Study the drawing (mm; zero at the part's minimum x, y, z) and answer. Coordinates: 2 decimals unless noted, no trailing zeros. Order: outer loops, then holes, each group sorted by start corner. A loop starts at its lowest first (then second) coordinate and runs counter-clockwise, first axis right, second up. Notation, with made-up numbers: (-3, 23) - (45, 23) arc R19 ccw to (45, 46) - close; hole circle Ø5 at (18, 55). An arc over 180 degrees is marked (long way). Write item = value, one per line.
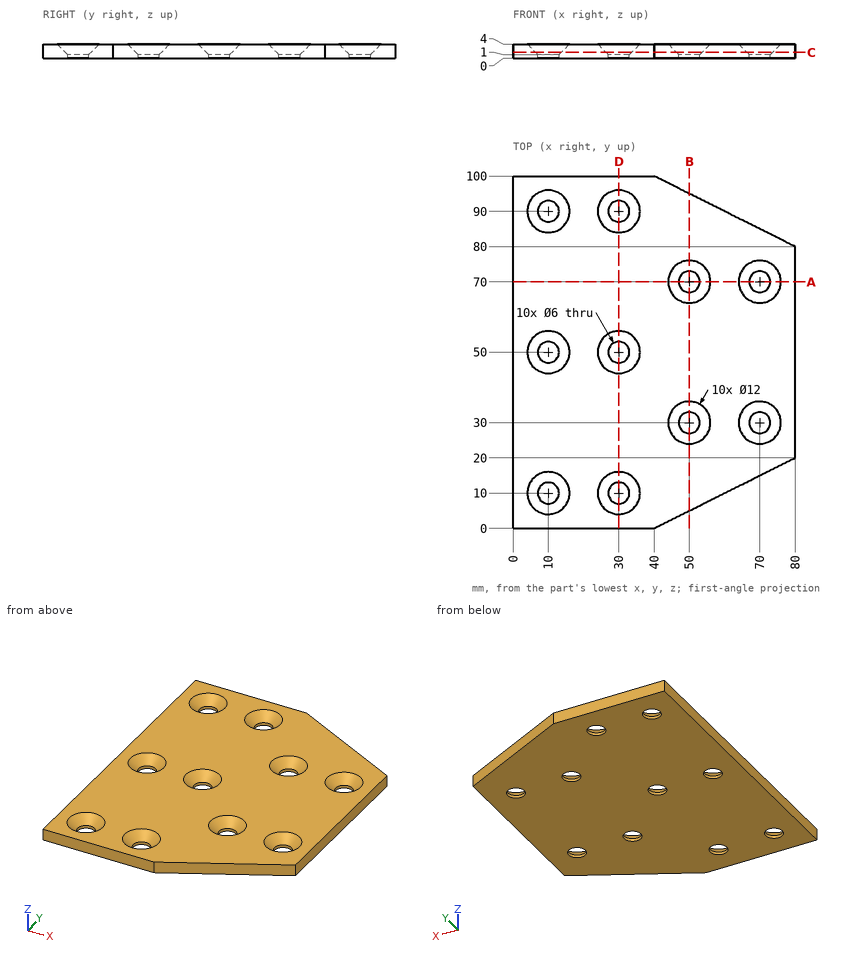
1) The part is cut by section A-A (y = 70). Determine the outline of the cut face in (x, z), and give its area (3 significant figures).
Returned:
outline = (0, 0) - (47, 0) - (47, 1) - (44, 4) - (0, 4) - close; (53, 0) - (67, 0) - (67, 1) - (64, 4) - (56, 4) - (53, 1) - close; (73, 0) - (80, 0) - (80, 4) - (76, 4) - (73, 1) - close
area = 254 mm^2
2) The part is cut by section B-B (x = 50). Determine the outline of the cut face in (y, z), and give its area (3 significant figures).
Returned:
outline = (5, 0) - (27, 0) - (27, 1) - (24, 4) - (5, 4) - close; (33, 0) - (67, 0) - (67, 1) - (64, 4) - (36, 4) - (33, 1) - close; (73, 0) - (95, 0) - (95, 4) - (76, 4) - (73, 1) - close
area = 294 mm^2
3) The part is cut by section C-C (z = 1.65). Count the separate pieces of the cut face and the enclosed holes in it, and give its area (3 significant figures).
Returned:
separate_pieces = 1
enclosed_holes = 10
area = 6,780 mm^2
4) Straight lines are drawn through the part: line 1 along Y through (x, z) = (30, 0.7); line 2 along Y through (x, z) = (29, 0.85); line 3 along X through (y, z) = (27, 3.8). For each, find the intervals that lie inside material, in ascending order. Write a range as from..to.
Returned:
line_1 = 0..7, 13..47, 53..87, 93..100
line_2 = 0..7.17, 12.83..47.17, 52.83..87.17, 92.83..100
line_3 = 0..45.04, 54.96..65.04, 74.96..80
5) Flat-ended cylindrical pins translate along their axes: pin 1 Ø5 at (x, y) = (30, 10) entering from +Z; pin 2 Ø8 at (x, y) = (10, 10) entering from +Z; pin 3 Ø7 at (x, y) = (70, 70) entering from +Z; pin 4 Ø9.5 at (x, y) = (30, 50) entering from +Z. Find the tip coordinate at first contact, or state that the pin passes through.
Returned:
pin_1 = through
pin_2 = 2
pin_3 = 1.5
pin_4 = 2.75
6) The part is cut by section D-D (x = 30). Determine the outline of the cut face in (y, z), and give its area (3 significant figures).
Returned:
outline = (0, 0) - (7, 0) - (7, 1) - (4, 4) - (0, 4) - close; (13, 0) - (47, 0) - (47, 1) - (44, 4) - (16, 4) - (13, 1) - close; (53, 0) - (87, 0) - (87, 1) - (84, 4) - (56, 4) - (53, 1) - close; (93, 0) - (100, 0) - (100, 4) - (96, 4) - (93, 1) - close
area = 301 mm^2
